from build123d import *

# Parameters (mm, degrees)
SKETCH2_R           = 3.5
BOSS_EXTRUDE1_DEPTH = 68.75
SKETCH3_R           = 5
BOSS_EXTRUDE2_DEPTH = 57.75
FILLET1_R           = 1


with BuildPart() as part:
    # Sketch1 → Revolve1 (revolve)
    with BuildSketch(Plane(origin=(0, 0, 0), x_dir=(1, 0, 0), z_dir=(0, 1, 0))):
        with BuildLine():
            Line((0, 5), (0, -5))
            ThreePointArc((0, -5), (5, 0), (0, 5))
        make_face()
    revolve(axis=Axis((0, 0, -5), (0, 0, 1)))

    # Sketch2 → Boss-Extrude1 (add)
    with BuildSketch(Plane(origin=(0, 0, 0), x_dir=(0, 0, -1), z_dir=(1, 0, 0))):
        with Locations(Location((0, 0, 0), (0, 0, 180))):
            Circle(SKETCH2_R)
    extrude(amount=BOSS_EXTRUDE1_DEPTH)

    # Sketch3 → Boss-Extrude2 (add)
    with BuildSketch(Plane(origin=(68.75, 0, 0), x_dir=(0, 0, -1), z_dir=(1, 0, 0))):
        Circle(SKETCH3_R)
    extrude(amount=-BOSS_EXTRUDE2_DEPTH)

    # Fillet1
    fillet1_edges = [part.edges().sort_by_distance(p)[0] for p in [
        (11, 0, 5),
    ]]
    fillet(fillet1_edges, radius=FILLET1_R)

    # Mirror1: part across face


with BuildPart() as part_1:
    add(part.part)
    add(part.part.mirror(Plane(origin=(68.75, 0, 0), x_dir=(0, 0, 1), z_dir=(1, 0, 0))))


solid = part_1.part
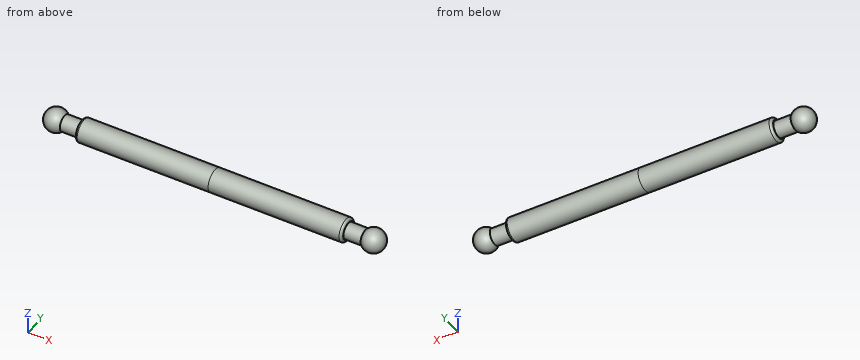
Could you check a few things on this model? Use its own coordinates, in mm. Give positions to 0.01 mm unless a question says otherwise; leave off trailing zeros. Order: outer loops, then holes, each group sorted by start corner. A loop starts at its lowest first (then second) coordinate and runs counter-clockwise, first axis right, second up.
1. For pin 1 (1.5 mm diameter, centred on y = -2, z = -2, fed in from -X); pin 2 (1 mm diameter, centred on y = 0.5, z = -3, fed in from -X); pin 3 (5 mm diameter, centred on y = 3, z = -1.5, fed in from +X), each with a flat end and sliding along its axis, tell me the tip position at first contact or that it passes through.
Answers below:
pin 1: stops at x = -4.55
pin 2: stops at x = -4.31
pin 3: stops at x = 142.43
2. I need wall thicknesses on L1, parallel to X at y = -4.5, z = 0.25; L2, parallel to X at y = 4, z = 0; L3, parallel to Y at x = 35, z = -0.25. Which ranges of each line are inside material? Lowest first, please.
Answers below:
L1: x = -2.17 to 2.17, 11.14 to 126.36, 135.33 to 139.67
L2: x = -3 to 3, 11 to 126.5, 134.5 to 140.5
L3: y = -4.99 to 4.99
3. Suppose I cut it at A-A (z = 0). Write out the boundary of the cut face in (x, y), plus the area to 3 significant figures.
Answers below:
outline: (3.57, -3.5) - (11, -3.5) - (11, -4) arc R1 ccw to (12, -5) - (125.5, -5) arc R1 ccw to (126.5, -4) - (126.5, -3.5) - (133.93, -3.5) arc R5 ccw (long way) to (133.93, 3.5) - (126.5, 3.5) - (126.5, 4) arc R1 ccw to (125.5, 5) - (12, 5) arc R1 ccw to (11, 4) - (11, 3.5) - (3.57, 3.5) arc R5 ccw (long way) to start
area: 1,400 mm2
4. Suppose I cut it at C-C (x = 59). Write out the boundary of the cut face in (y, z), plus the area to 3 significant figures.
Answers below:
outline: circle Ø10 at (0, 0)
area: 78.5 mm2
